Could you check a few things on this model? Use its own coordinates, in mm. Face numbers are marked on the shaded views. Give positions to 0.01 mm unless a question says otherwise; leave off trailing zeros. Loops run counter-clockwise (first coordinate to the right, second up) from the corner with the lowest first, then second, coordinate; pieces in that order, holes last. Notation, with made-up numbers: M 69,84 L 124,84 A11 cw 124,93 Z; hole C -3.75,48.25 d8. An arc over 180 degrees is marked long. Answer in a Markdown table with one row per item. Add a question column.
1. I'm going to push flat-ended pins straight in: pin 1 Ø8 at (y, z) = (6, -117.5) entering from +X; pin 2 Ø3 at (y, z) = (22, -32.5) entering from -X; pin 3 Ø6 at (x, y) = (187.5, 12.5) entering from +Z; pin 4 Ø10 at (x, z) = (177, -102.5) entering from -Y. Where does each tip first touch, or does it pass through?
2. If we section it at A-A on y = 14.5: List the corners of the cut face in (x, z) for me (1 decimal).
3. If we section it at B-B on x = 198: List the corners of the cut face in (y, z) for me, then the cut area to 3 significant figures.
4. Thinking about a two-plate mould opening in Z: for the marked faces 1 and 2, which applies, released by +Z, released by -Z, zero draft, split by the parting line, or undercut?
5. I need wall thicknesses on line 1 along Z through (x, y) = (174, 12); line 2 along X through (y, z) = (23, -115.5); line 3 along Z through (x, y) = (175.5, 18.5). Which ranges of each line are inside material? Lowest first, please. Write a range as from..to.
6. If we section it at C-C on y = 3: List the corners of the cut face in (x, z) for me (3 decimals).
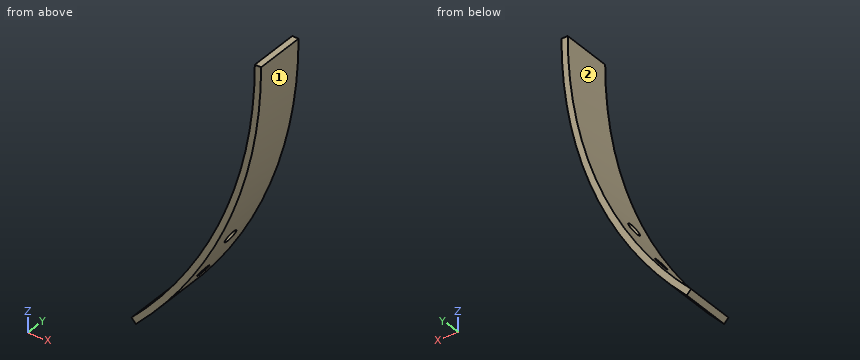
Autodesk Inventor part; units mm, degrees
ref_plane "YZ Plane" through (0, 0, 0) normal (1, 0, 0) x (0, 1, 0)
ref_plane "XZ Plane" through (0, 0, 0) normal (0, 1, 0) x (-1, 0, 0)
ref_plane "XY Plane" through (0, 0, 0) normal (0, 0, 1) x (1, 0, 0)
sketch "Sketch1" plane through (0, 0, 0) normal (0, 1, 0) x (-1, 0, 0)
  arc A0 (-215.9, 0) -> (-152.6644, -152.6644) centre (0, 0) ccw
  arc A1 (-212.725, 0) -> (-150.4193, -150.4193) centre (0, 0) ccw
  line L0 (-150.4193, -150.4193) -> (-152.6644, -152.6644)
  line L1 (-212.725, 0) -> (-215.9, 0)
  dimension "d0" = 431.8
  dimension "d1" = 3.175
  dimension "d2" = 45
extrude "Extrusion1" add sketch "Sketch1" along normal blind 25.4
ref_plane "Work Plane1" through (152.6644, 0, -152.6644) normal (0.7071, 0, -0.7071) x (0, 1, 0)
sketch "Sketch2" plane through (152.6644, 0, -152.6644) normal (0.7071, 0, -0.7071) x (0, 1, 0)
  circle A0 centre (12.7, 38.1) radius 3.3734
  line L0 (0, 0) -> (25.4, 0)
  circle A1 centre (12.7, 63.8969) radius 3.3734
  line L1 (25.4, 150.4193) -> (25.4, 0)
  dimension "d5" = 6.7469
  dimension "d6" = 38.1
  dimension "d7" = 6.7469
  dimension "d8" = 19.05
  dimension "d9" = 12.7
  dimension "d10" = 12.7
extrude "Extrusion2" cut sketch "Sketch2" against normal blind 17.78
properties material "Aluminum 6061"
Results:
| question | item | result |
|---|---|---|
| 1 | pin 1 | x = 183.66 |
| 1 | pin 2 | x = 209.99 |
| 1 | pin 3 | z = -94.67 |
| 1 | pin 4 | through |
| 2 | outline | M 150.4,-150.4 L 152.7,-152.7 A215.9 ccw 175.5,-125.7 L 173.3,-123.4 A212.7 cw Z; M 176.6,-118.6 L 178.9,-120.9 A215.9 ccw 189.6,-103.3 L 187.3,-100.9 A212.7 cw Z; M 190,-95.6 L 192.4,-98 A215.9 ccw 215.9,0 L 212.7,0 A212.7 cw Z |
| 3 | outline | M 0,-86.07 L 25.4,-86.07 L 25.4,-77.77 L 0,-77.77 Z |
| 3 | area | 211 mm2 |
| 4 | face 1 | released by -Z |
| 4 | face 2 | released by +Z |
| 5 | line 1 | -127.82..-124.79 |
| 5 | line 2 | 178.64..182.41 |
| 5 | line 3 | -125.75..-120.22 |
| 6 | outline | M 150.419,-150.419 L 152.664,-152.664 A215.9 ccw 215.9,0 L 212.725,0 A212.725 cw Z |
